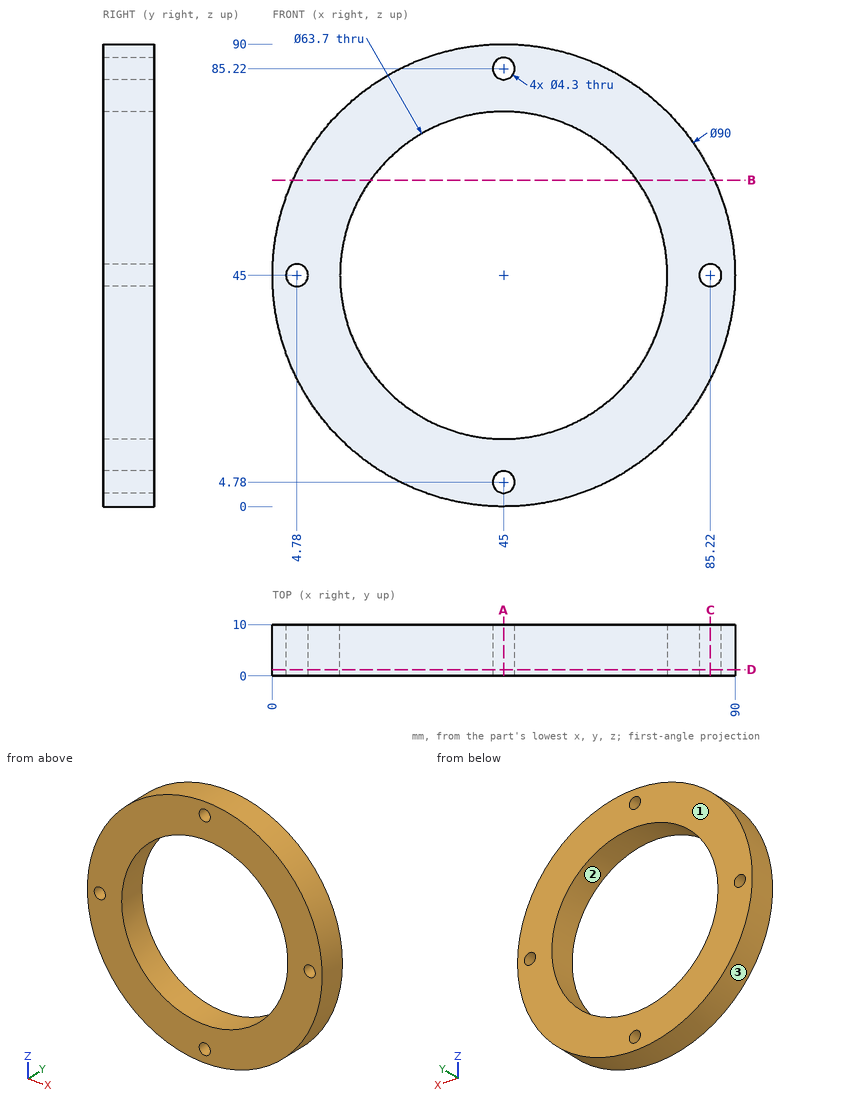
Geometry: see drawing. Coordinates: mm, zero at the bounding-box minimum. Round coordinates to 2 decimals unless told otherwise and drop trailing zeros. Write each loop counter-clockwise with the first axis right and the second up, starting at its lowest first coordinate (ties: lowest second). Pieces come first, ordered by that corner, then holes. Notation, with made-up numbers: (27.25, 50) - (63.25, 50) arc R14 ccw to (63.25, 71) - close; hole circle Ø5 at (-3.75, 69.25). An arc over 180 degrees is marked (long way). Use CSV: the item, a comma, the result in double quotes. Start each with the question number.
(1) Mould query, pull axis Z, two halves, no side actions, for the marked faces 1, 2 and 3. Classes: pulls with the +Z half, pulls with the -Z half, needs draft (parallel to the pull), parting line crosses it, or undercut.
(2) Material intervals for probe 1 along Z at (x, y) = (45, 8.25); probe 2 along Z at (x, y) = (63, 6.5); probe 3 along Z at (x, y) = (36, 9.75), sorted ascending. Write a range as [from, to].
(3) Cut plane C-C, the plane x = 85.22. Return loops of the section in (y, z), and give its area (3 significant figures).
(4) Cut plane A-A, the plane x = 45. Return loops of the section in (y, z), and give its area (3 significant figures).
(5) First-contact query: pin 1 Ø4 at (x, z) = (45, 85.22) entering from +Y; pin 2 Ø5 at (x, y) = (27.5, 6.5) entering from -Z; pin 3 Ø2 at (x, y) = (16, 1) entering from -Z. Flat tips, straight axial feed; report the tip coordinate or a pass-through.
(6) Cut plane D-D, the plane y = 1.25. Return loops of the section in (x, z), and give its area (3 significant figures).
(7) Cut plane B-B, the plane z = 63.5. Return loops of the section in (x, y).
Geometry says:
1,face 1,"needs draft"
1,face 2,"undercut"
1,face 3,"parting line crosses it"
2,probe 1,"[0, 2.63], [6.93, 13.15], [76.85, 83.07], [87.37, 90]"
2,probe 2,"[3.76, 18.72], [71.28, 86.24]"
2,probe 3,"[0.91, 14.45], [75.55, 89.09]"
3,outline,"(0, 24.82) - (10, 24.82) - (10, 42.85) - (0, 42.85) - close; (0, 47.15) - (10, 47.15) - (10, 65.18) - (0, 65.18) - close"
3,area,"361 mm²"
4,outline,"(0, 0) - (10, 0) - (10, 2.63) - (0, 2.63) - close; (0, 6.93) - (10, 6.93) - (10, 13.15) - (0, 13.15) - close; (0, 76.85) - (10, 76.85) - (10, 83.07) - (0, 83.07) - close; (0, 87.37) - (10, 87.37) - (10, 90) - (0, 90) - close"
4,area,"177 mm²"
5,pin 1,"through"
5,pin 2,"z = 2.57"
5,pin 3,"z = 9.77"
6,outline,"circle Ø90 at (45, 45); hole circle Ø4.3 at (4.78, 45); hole circle Ø63.7 at (45, 45); hole circle Ø4.3 at (45, 4.78); hole circle Ø4.3 at (45, 85.22); hole circle Ø4.3 at (85.22, 45)"
6,area,"3,120 mm²"
7,outline,"(3.98, 0) - (19.07, 0) - (19.07, 10) - (3.98, 10) - close; (70.93, 0) - (86.02, 0) - (86.02, 10) - (70.93, 10) - close"
